Source: CAD feature listing. Evaluate the final solid. Frame: model axes, mm. A direction names the side the tool comes from. Round coordinates to 2 decimals unless told otherwise and drop trailing zeros. Write each loop counter-clockwise with the first axis right and the second up, starting at its lowest first coordinate (ties: lowest second). Pieces come first, ordered by that corner, then holes. Notation, with made-up numbers: (87, 39.5) -> (106, 39.5) arc R21 cw to (106, 50.5) -> close; hole circle Ø9 at (-1, -15.5). An arc over 180 degrees is marked (long way). Put each result on its own line as item: value.
```python
from build123d import *

# Parameters (mm, degrees)
SKETCH_1_R          = 35
EXTRUDE_1_DEPTH     = 3
SKETCH_2_R          = 27.4
EXTRUDE_2_DEPTH     = 6
SKETCH_3_R          = 1.6
CUT_EXTRUDE_1_DEPTH = 51.309044912
SKETCH_4_R          = 15
CUT_EXTRUDE_2_DEPTH = 51.309044912
SKETCH_5_R          = 1.25
CUT_EXTRUDE_3_DEPTH = 51.309044912


with BuildPart() as part:
    # ｽｹｯﾁ1 → ﾎﾞｽ - 押し出し1 (new body)
    with BuildSketch(Plane(origin=(0, 0, 0), x_dir=(1, 0, 0), z_dir=(0, 1, 0))):
        with Locations(Location((0, 0, 0), (0, 0, 270))):
            Circle(SKETCH_1_R)
    extrude(amount=EXTRUDE_1_DEPTH)

    # ｽｹｯﾁ2 → ﾎﾞｽ - 押し出し2 (add)
    with BuildSketch(Plane(origin=(0, 3, 0), x_dir=(1, 0, 0), z_dir=(0, 1, 0))):
        with Locations(Location((0, 0, 0), (0, 0, 270))):
            Circle(SKETCH_2_R)
    extrude(amount=EXTRUDE_2_DEPTH)

    # ｽｹｯﾁ3 → ｶｯﾄ - 押し出し1 (cut, through all)
    with BuildSketch(Plane(origin=(0, 9, 0), x_dir=(1, 0, 0), z_dir=(0, 1, 0))):
        with Locations(Location((0, 20, 0), (0, 0, 270))):
            Circle(SKETCH_3_R)
        with Locations(Location((20, 0, 0), (0, 0, 270))):
            Circle(SKETCH_3_R)
        with Locations(Location((0, -20, 0), (0, 0, 270))):
            Circle(SKETCH_3_R)
        with Locations(Location((-20, 0, 0), (0, 0, 270))):
            Circle(SKETCH_3_R)
    extrude(amount=-CUT_EXTRUDE_1_DEPTH, mode=Mode.SUBTRACT)

    # ｽｹｯﾁ4 → ｶｯﾄ - 押し出し2 (cut, through all)
    with BuildSketch(Plane(origin=(0, 9, 0), x_dir=(1, 0, 0), z_dir=(0, 1, 0))):
        with Locations(Location((0, 0, 0), (0, 0, 270))):
            Circle(SKETCH_4_R)
    extrude(amount=-CUT_EXTRUDE_2_DEPTH, mode=Mode.SUBTRACT)

    # ｽｹｯﾁ5 → ｶｯﾄ - 押し出し3 (cut, through all)
    with BuildSketch(Plane.XZ):
        with Locations(Location((-14.142135624, 14.142135624, 0), (0, 0, 270))):
            Circle(SKETCH_5_R)
        with Locations(Location((14.142135624, 14.142135624, 0), (0, 0, 270))):
            Circle(SKETCH_5_R)
        with Locations(Location((14.142135624, -14.142135624, 0), (0, 0, 270))):
            Circle(SKETCH_5_R)
        with Locations(Location((-14.142135624, -14.142135624, 0), (0, 0, 270))):
            Circle(SKETCH_5_R)
    extrude(amount=-CUT_EXTRUDE_3_DEPTH, mode=Mode.SUBTRACT)


solid = part.part
```
Q1. Cut plane D-D on y = 4.5. Give the number of separate pieces and of enclosed holes in the cut face, and give its area (3 significant figures).
Ans:
separate pieces: 1
enclosed holes: 9
area: 1,600 mm^2
Q2. Reachability of faces 1 (the flat face through (-18, 3, -21)), 2 (the cylindrical face through (15.381, 4.437, 14.305)) from +Z, -Z, +X, -X, +Y, -Y: full face, straight path, thin tool, end or side. Return the list, or none.
Ans:
face 1: +Y
face 2: +Y, -Y
Q3. Cut plane A-A on x = 0. Output: boundary loops of the cut face in (y, z), and give its area (3 significant figures).
Ans:
outline: (0, -35) -> (3, -35) -> (3, -27.4) -> (9, -27.4) -> (9, -21.6) -> (0, -21.6) -> close; (0, -18.4) -> (9, -18.4) -> (9, -15) -> (0, -15) -> close; (0, 15) -> (9, 15) -> (9, 18.4) -> (0, 18.4) -> close; (0, 21.6) -> (9, 21.6) -> (9, 27.4) -> (3, 27.4) -> (3, 35) -> (0, 35) -> close
area: 211 mm^2
Q4. Pin query (flat end, axial travel): pin 1 (2 mm diameter, centred on x = -9.5, y = 3.5, fed in from -Z); pin 2 (3 mm diameter, centred on y = 6, z = 21, fed in from +X); pin 3 (3 mm diameter, centred on y = 7, z = -15, fed in from +X). Return the tip coordinate at first contact, or that it passes through.
Ans:
pin 1: stops at z = -33.92
pin 2: stops at x = 19.25
pin 3: stops at x = 23.84
Q5. Material intervals for line 1 (X direction, y = 3.25, z = 0); line 2 (Z direction, x = -1, y = 2.75); line 3 (X direction, y = 3.75, z = 19), sorted ascending. Write a range as [from, to].
Ans:
line 1: x = [-27.4, -21.6], [-18.4, -15], [15, 18.4], [21.6, 27.4]
line 2: z = [-34.99, -21.25], [-18.75, -14.97], [14.97, 18.75], [21.25, 34.99]
line 3: x = [-19.74, -1.25], [1.25, 19.74]
Q6. Draft query along X for faces 3 (the flat face through (-7, 0, 15)), 4 (the cylindrical face through (-18.414, 4.563, -0.208)), 5 (the cylindrical face through (8.23, 5.958, 26.135)). Return one class per face: +X half, -X half, draft (parallel to the pull), parting line (faces both ways), or undercut.
Ans:
face 3: draft
face 4: undercut
face 5: parting line
Q7. Cut plane B-B on z = 0. Output: boundary loops of the cut face in (x, y).
Ans:
outline: (-35, 0) -> (-21.6, 0) -> (-21.6, 9) -> (-27.4, 9) -> (-27.4, 3) -> (-35, 3) -> close; (-18.4, 0) -> (-15, 0) -> (-15, 9) -> (-18.4, 9) -> close; (15, 0) -> (18.4, 0) -> (18.4, 9) -> (15, 9) -> close; (21.6, 0) -> (35, 0) -> (35, 3) -> (27.4, 3) -> (27.4, 9) -> (21.6, 9) -> close
Q8. Cut plane C-C on z = -20. Output: boundary loops of the cut face in (x, y), and give its area (3 significant figures).
Ans:
outline: (-28.72, 0) -> (-1.6, 0) -> (-1.6, 9) -> (-18.73, 9) -> (-18.73, 3) -> (-28.72, 3) -> close; (1.6, 0) -> (28.72, 0) -> (28.72, 3) -> (18.73, 3) -> (18.73, 9) -> (1.6, 9) -> close
area: 368 mm^2
